The model under review builds one solid part; all positions refer to its coordinate system, in mm. Face numbers are marked on the shaded views. A direction names the side the tool comes from. Round coordinates to 2 decimals unless told otherwise and drop trailing zeros. Order: outer loops, then holes, each group sorted by start corner. A loop starts at its lowest first (then second) coordinate and runs counter-clockwise, first axis right, second up.
1) Consider section C-C (x = 1). Give the boundary of the cut face in (y, z).
2) Consider section B-B (y = 6.5). Give the boundary of the cut face in (x, z).
3) To check wall thickness, follow L1, parallel to Y at x = -10, z = 2; L2, parallel to Z at x = -0.5, y = 0; L3, parallel to X at y = -17, z = 31. State the ranges of each line that lie inside material, in increasing order.
4) Machinability: for the marked faces 1, 2 and 3, which of the approach directions +Z, -Z, +X, -X, +Y, -Y give a long, thin tool a straight path to every point of the face, cutting with its end or side? Answer none if there is none.
5) Consider section A-A (z = 30). Give the boundary of the cut face in (x, y).
6) Consider section D-D (y = -17.5). Give the boundary of the cut face in (x, z), then the cut area to 3 significant figures.
7) Mouldability with a two-part tool opening along X and no side actions: class the marked faces 4, 5 and 6 as pulls with the +X half, pulls with the -X half, needs draft (parallel to the pull), parting line crosses it, or undercut.
8) Clearance check with flat-ended pins moving along their axes: P1, Ø4, axis at x = 10, y = -6.5, coming from the -Z side; P2, Ø13, axis at x = 5, z = -28, coming from the -Y side; P3, Ø22.5, axis at x = 8, y = 18, coming from the -Z side. State where each tip first meets the part, or that it passes through.
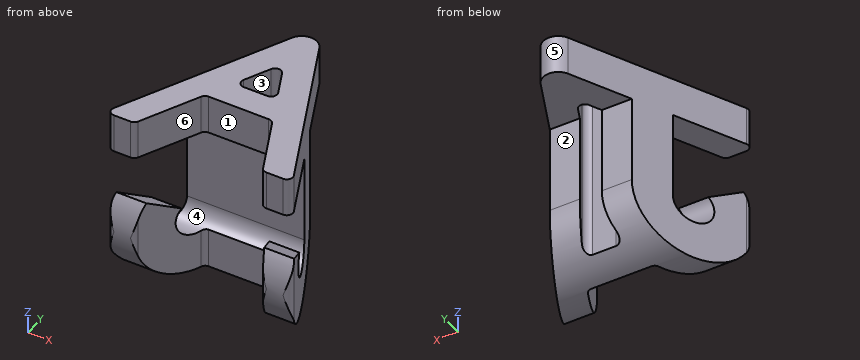
from build123d import *

# Parameters (mm, degrees)
F1_DEPTH = 38.1
F4_DEPTH = 63.5


with BuildPart() as f1:
    # F0 (on Top) → F1 (new body, symmetric)
    with BuildSketch(Plane.XY):
        with BuildLine():
            Line((37.8624187806, -34.487401399), (5.7560469514, 34.4314965026))
            ThreePointArc((5.7560469514, 34.4314965026), (0, 38.1), (-5.7560469514, 34.4314965026))
            Line((-5.7560469514, 34.4314965026), (-37.8624187806, -34.487401399))
            ThreePointArc((-37.8624187806, -34.487401399), (-37.7019617698, -36.9251372739), (-35.56, -38.1))
            Line((-35.56, -38.1), (-28.5547583227, -38.1))
            ThreePointArc((-28.5547583227, -38.1), (-27.1896210488, -37.7019617698), (-26.2523395422, -36.632598601))
            Line((-26.2523395422, -36.632598601), (-14.9362832259, -12.3417776368))
            ThreePointArc((-14.9362832259, -12.3417776368), (-13.9990017193, -11.2724144681), (-12.6338644453, -10.8743762379))
            Line((-12.6338644453, -10.8743762379), (12.6338644453, -10.8743762379))
            ThreePointArc((12.6338644453, -10.8743762379), (13.9990017193, -11.2724144681), (14.9362832259, -12.3417776368))
            Line((14.9362832259, -12.3417776368), (26.2523395422, -36.632598601))
            ThreePointArc((26.2523395422, -36.632598601), (27.1896210488, -37.7019617698), (28.5547583227, -38.1))
            Line((28.5547583227, -38.1), (35.56, -38.1))
            ThreePointArc((35.56, -38.1), (37.7019617698, -36.9251372739), (37.8624187806, -34.487401399))
        make_face()
        with BuildLine():
            ThreePointArc((-2.3024187806, 14.7778239937), (0, 16.2452253927), (2.3024187806, 14.7778239937))
            Line((2.3024187806, 14.7778239937), (7.2449791708, 4.1682223632))
            ThreePointArc((7.2449791708, 4.1682223632), (7.0845221601, 1.7304864882), (4.9425603903, 0.5556237621))
            Line((4.9425603903, 0.5556237621), (-4.9425603903, 0.5556237621))
            ThreePointArc((-4.9425603903, 0.5556237621), (-7.0845221601, 1.7304864882), (-7.2449791708, 4.1682223632))
            Line((-7.2449791708, 4.1682223632), (-2.3024187806, 14.7778239937))
        make_face(mode=Mode.SUBTRACT)
    extrude(amount=F1_DEPTH, both=True)

    # F3 (on Right) → F4 (intersect, symmetric)
    with BuildSketch(Plane.YZ):
        with BuildLine():
            Line((38.1, 38.1), (-38.1, 38.1))
            Line((-38.1, 38.1), (-38.1, 22.0156293362))
            Line((-38.1, 22.0156293362), (-6.1763821984, 22.0156293362))
            Line((-6.1763821984, 22.0156293362), (-6.1763821984, -14.164009311))
            ThreePointArc((-6.1763821984, -14.164009311), (-17.2167607386, -21.5452622947), (-19.8182046927, -8.5220006727))
            Line((-19.8182046927, -8.5220006727), (-33.4594100714, 0))
            ThreePointArc((-33.4594100714, 0), (-21.6164289624, -36.9102857448), (9.7719813781, -14.164009311))
            Line((9.7719813781, -14.164009311), (9.7719813781, 22.0156293362))
            Line((9.7719813781, 22.0156293362), (38.1, 22.0156293362))
            Line((38.1, 22.0156293362), (38.1, 38.1))
        make_face()
    extrude(amount=F4_DEPTH, both=True, mode=Mode.INTERSECT)


solid = f1.part
Answer below:
1. outline: (-10.87, -37.87) arc R23.94 ccw to (0.56, -33.04) - (0.56, 38.1) - (-10.87, 38.1) - (-10.87, 22.02) - (-6.18, 22.02) - (-6.18, -14.16) arc R7.99 cw to (-10.87, -21.44) - close; (16.04, 22.02) - (38.02, 22.02) - (38.02, 38.1) - (16.04, 38.1) - close
2. outline: (-18.77, -26.24) - (-6.16, -26.24) - (-6.16, 38.1) - (-18.77, 38.1) - close; (6.16, -26.24) - (18.77, -26.24) - (18.77, 38.1) - (6.16, 38.1) - close
3. L1: y = -6.18 to 9.77
3. L2: z = -33.46 to 38.1
3. L3: x = -29.72 to -17.11, 17.11 to 29.72
4. face 1: +Z, -Z, -Y
4. face 2: -Z, +X, -X, +Y
4. face 3: +Z, -Z
5. outline: (-37.86, -34.49) arc R2.54 ccw to (-35.56, -38.1) - (-28.55, -38.1) arc R2.54 ccw to (-26.25, -36.63) - (-14.94, -12.34) arc R2.54 cw to (-12.63, -10.87) - (12.63, -10.87) arc R2.54 cw to (14.94, -12.34) - (26.25, -36.63) arc R2.54 ccw to (28.55, -38.1) - (35.56, -38.1) arc R2.54 ccw to (37.86, -34.49) - (5.76, 34.43) arc R6.35 ccw to (-5.76, 34.43) - close; hole (-7.24, 4.17) arc R2.54 ccw to (-4.94, 0.56) - (4.94, 0.56) arc R2.54 ccw to (7.24, 4.17) - (2.3, 14.78) arc R2.54 ccw to (-2.3, 14.78) - close
6. outline: (-29.95, -37.87) - (-17.34, -37.87) - (-17.34, -21.42) - (-29.95, -21.42) - close; (-29.95, 22.02) - (-17.34, 22.02) - (-17.34, 38.1) - (-29.95, 38.1) - close; (17.34, -37.87) - (29.95, -37.87) - (29.95, -21.42) - (17.34, -21.42) - close; (17.34, 22.02) - (29.95, 22.02) - (29.95, 38.1) - (17.34, 38.1) - close
6. area: 820 mm2
7. face 4: needs draft
7. face 5: parting line crosses it
7. face 6: undercut
8. P1: stops at z = -37.42
8. P2: stops at y = -10.87
8. P3: stops at z = -25.81
